Autodesk Inventor part; units mm, degrees
ref_plane "YZ Plane" through (0, 0, 0) normal (1, 0, 0) x (0, 1, 0)
ref_plane "XZ Plane" through (0, 0, 0) normal (0, 1, 0) x (-1, 0, 0)
ref_plane "XY Plane" through (0, 0, 0) normal (0, 0, 1) x (1, 0, 0)
sketch "Sketch1" plane through (0, 0, 0) normal (0, 0, 1) x (1, 0, 0)
  circle A0 centre (0, 0) radius 10
  circle A1 centre (0, 0) radius 12.5
  dimension "d0" = 0
  dimension "d1" = 0
  dimension "d2" = 0
  dimension "d3" = 0
  dimension "d4" = 25
  dimension "d5" = 20
extrude "Extrusion1" add sketch "Sketch1" along normal blind 10
extrude "Extrusion2" add sketch "Sketch1" against normal blind 29 contours A0
sketch "Sketch2" plane through (0, 0, -29) normal (0, 0, -1) x (-1, 0, 0)
  circle A0 centre (0, 0) radius 8.5
  dimension "d10" = 17
extrude "Extrusion3" add sketch "Sketch2" along normal blind 1
sketch "Sketch3" plane through (0, 0, -30) normal (0, 0, -1) x (-1, 0, 0)
  circle A0 centre (0, 0) radius 3
  dimension "d13" = 6
extrude "Extrusion4" add sketch "Sketch3" along normal blind 6
thread "Thread1"
sketch "Sketch4" plane through (0, 0, 10) normal (0, 0, 1) x (1, 0, 0)
  circle A0 centre (0, 0) radius 10
  line L0 (-10, 0) -> (-10, 2)
  line L1 (-10, 2) -> (-12.8956, 2)
  line L2 (-10, 0) -> (-11.1456, 0)
  line L3 (-10, 0) -> (-10, -2)
  line L4 (-10, -2) -> (-12.8956, -2)
  line L5 (-12.8956, -2) -> (-12.8956, 2)
extrude "Extrusion5" cut sketch "Sketch4" against normal up to surface (10 mm away) contours L3 L4 L5 L1 L0
sketch "Sketch5" plane through (0, 0, 0) normal (0, 0, 1) x (1, 0, 0)
  circle A0 centre (0, 0) radius 10
  circle A1 centre (0, 0) radius 8.5
  point P0 (-10, 0)
extrude "Extrusion6" add sketch "Sketch5" along normal blind 10
properties part number "piraki"
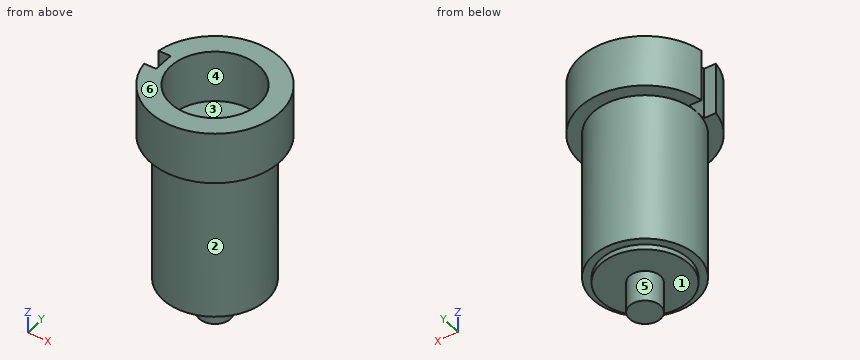
Geometry: final body of the model. Coordinates: model frame, mm. Face numbers are marked on the shaded views. A direction names the side the tool comes from. Give positions to 0.01 mm unless a question says otherwise; leave off trailing zeros. Order: outer loops, then holes, each group sorted by start corner. A loop starts at its lowest first (then second) coordinate and runs counter-clockwise, first axis right, second up. Notation, with made-up numbers: (84.5, -19) - (114.5, -19) arc R5 ccw to (114.5, -12) - close; hole circle Ø2 at (58, 0). An arc over 180 degrees is marked (long way). Use CSV: the item, a comma, the result in double quotes.
1. Mould query, pull axis Y, two halves, no side actions, for the marked faces 1, 2, 3 and 4. Classes: +Y half, -Y half, draft (parallel to the pull), parting line (faces both ways), or undercut.
Answers below:
face 1,"draft"
face 2,"parting line"
face 3,"undercut"
face 4,"undercut"
2. Section query C-C (y = -7.5). Output: boundary loops of the cut face in (x, z).
Answers below:
outline,"(-10, 0) - (-6.61, 0) - (-6.61, -29) - (-4, -29) - (-4, -30) - (4, -30) - (4, -29) - (6.61, -29) - (6.61, 0) - (10, 0) - (10, 10) - (4, 10) - (4, 0) - (-4, 0) - (-4, 10) - (-10, 10) - close"
3. Section query B-B (x = 0). Output: boundary loops of the cut face in (y, z).
Answers below:
outline,"(-12.5, 0) - (-10, 0) - (-10, -29) - (-8.5, -29) - (-8.5, -30) - (-3, -30) - (-3, -36) - (3, -36) - (3, -30) - (8.5, -30) - (8.5, -29) - (10, -29) - (10, 0) - (12.5, 0) - (12.5, 10) - (8.5, 10) - (8.5, 0) - (-8.5, 0) - (-8.5, 10) - (-12.5, 10) - close"
4. Contact query for flat-ended pins moving along their axis: pin 1 (8 mm diameter, centred on x = 5.5, z = -12, fed in from -Y); pin 2 (5 mm diameter, centred on x = 3.5, y = -2.5, fed in from +Z); pin 3 (4 mm diameter, centred on x = -7, z = -17.5, fed in from -Y); pin 4 (7.5 mm diameter, centred on x = 5, y = -3, fed in from -Z). Output: stop coordinate, or through.
Answers below:
pin 1,"y = -9.89"
pin 2,"z = 0"
pin 3,"y = -8.66"
pin 4,"z = -36"
5. Section query A-A (z = 5). Output: boundary loops of the cut face in (x, y).
Answers below:
outline,"(-12.34, -2) arc R12.5 ccw (long way) to (-12.34, 2) - (-10, 2) - (-10, -2) - close; hole circle Ø17 at (0, 0)"
6. Section query D-D (z = -20). Output: boundary loops of the cut face in (x, y), plus the area to 3 significant figures.
Answers below:
outline,"circle Ø20 at (0, 0)"
area,"314 mm2"
7. Material intervals for line 1 along Y through (x, z) = (0, 7); line 2 along X through (y, z) = (0, -22.5); line 3 along Z through (x, y) = (-2.5, -3.25), sorted ascending. Write a range as from..to.
Answers below:
line 1,"-12.5..-8.5, 8.5..12.5"
line 2,"-10..10"
line 3,"-30..0"
8. Access query for the marked faces 5 and 6. Directions: +Z, -Z, +X, -X, +Y, -Y. A direction counts if a zero-diameter tool reaches every point of the face in a straight line with its end or side. Return the directions, or none.
Answers below:
face 5,"-Z"
face 6,"+Z, +X, -X, +Y, -Y"
